Autodesk Inventor part; units mm, degrees
ref_plane "Work Plane1" through (3, 0, 1) normal (0, 0, 1) x (1, 0, 0)
ref_plane "YZ Plane" through (0, 0, 0) normal (1, 0, 0) x (0, 1, 0)
ref_plane "XZ Plane" through (0, 0, 0) normal (0, 1, 0) x (-1, 0, 0)
sketch "Sketch1" plane through (0, 0, 0) normal (0, 1, 0) x (-1, 0, 0)
  line L0 (0, 0) -> (-6, 0)
  line L1 (-6, 0) -> (-6, -9)
  line L2 (-6, -9) -> (0, -9)
  line L3 (0, -9) -> (0, 0)
  dimension "d0" = 6
  dimension "d1" = 9
extrude "Extrusion1" add sketch "Sketch1" along normal blind 6
sketch "Sketch2" plane through (6, 0, -9) normal (0, 0, -1) x (-1, 0, 0)
  line L0 (0, 6) -> (6, 6)
  line L1 (0, 0) -> (6, 0)
  line L2 (1.5, 6) -> (4.5, 6)
  line L3 (4.5, 6) -> (4.5, 0)
  line L4 (4.5, 0) -> (1.5, 0)
  line L5 (1.5, 0) -> (1.5, 6)
  line L6 (0, 0) -> (0, 6)
  dimension "d4" = 3
  dimension "d5" = 1.5
sketch "Sketch3" plane through (0, 0, 0) normal (0, -1, 0) x (1, 0, 0)
  line L0 (6, 0) -> (6, -9)
  line L1 (0, 0) -> (6, 0)
  point P0 (3, 1)
  dimension "d6" = 3
  dimension "d7" = 1
ref_plane "Work Plane1" through (3, 0, 1) normal (0, 0, 1) x (1, 0, 0)
sketch "Sketch4" plane through (3, 0, 1) normal (0, 0, 1) x (1, 0, 0)
  point P0 (-3, 0)
sketch "Sketch5" plane through (3, 0, 1) normal (0, 0, 1) x (1, 0, 0)
  circle A0 centre (0, 3) radius 1.5
  point P0 (-3, 0)
  dimension "d8" = 3
loft "Loft1" add profiles "Sketch5" section 1 edges at (3, 0, 0) (6, 3, 0) (3, 6, 0) (0, 3, 0)
extrude "Extrusion2" cut sketch "Sketch2" against normal blind 7 contours L0 L3 L1 L5
sketch "Sketch6" plane through (6, 0, -9) normal (1, 0, 0) x (0, 0, -1)
  line L0 (-9, 0) -> (-9, 6)
  line L1 (-9, 6) -> (0, 6)
  point P0 (-3, 3)
  dimension "d15" = 6
  dimension "d16" = 3
hole "Hole1" at (6, 3, -6) direction (-1, 0, 0) diameter 2.5 depth 1.5 tip angle 118
sketch "Sketch7" plane through (0, 0, -9) normal (-1, 0, 0) x (0, 0, 1)
  circle A0 centre (3, 3) radius 1.25
  point P0 (9, 0)
hole "Hole2" at (0, 3, -6) at (0, 3, -6) direction (1, 0, 0) diameter 3 depth 1.5 tip angle 118
thread "Thread1"
fillet "Fillet1" radius 3 4 edges at (5.25, 6, -9) (5.25, 0, -9) (0.75, 0, -9) (0.75, 6, -9)
sketch "Sketch8" plane through (6, 0, -2) normal (0, 0, -1) x (-1, 0, 0)
  line L0 (4.5, 6) -> (4.5, 0)
  line L1 (1.5, 6) -> (4.5, 6)
  line L2 (1.5, 0) -> (1.5, 6)
  line L3 (4.5, 0) -> (1.5, 0)
  point P0 (6, 0)
  point P1 (3, 3)
properties material "Brass, Soft Yellow, Welded"
Input: part model. Units: mm. Frame: model coordinates. A direction names the side the tool comes from. Coordinates: 2 decimals unless noted, no trailing zeros. Order: outer loops, then holes, each group sorted by start corner. A loop starts at its lowest first (then second) coordinate and runs counter-clockwise, first axis right, second up. Notation, with made-up numbers: M -20.75,70 L -6.75,70 A24 ccw -6.75,97 Z; hole C 49,86.25 d5. An arc over 180 degrees is marked long. Write item = value, one per line. Start each with the question number.
(1) Line query: line 1 along X through (y, z) = (0.75, -5.75); line 2 along Y through (x, z) = (5.2, -6). Output: solid intervals per line, ascending. Write a range as [from, to].
(2) First-contact query: P1, Ø2, axis at y = 3, z = -6, coming from the +X side; P2, Ø1.5, axis at x = 3.5, y = 3, coming from the -Z side. Flat tips, straight axial feed; report the tip coordinate or a pass-through.
(3) Reachability of faces 5 (the flat face through (1.5, 3, -4)), 6 (the cylindrical face through (0.74, 0.9, -8.14)) from +Z, -Z, +X, -X, +Y, -Y: full face, straight path, thin tool, end or side. Return the list, or none.
(4) Pull-direction query (Y, two-part tool) for faces 1 (the cylindrical face through (5.24, 2.95, -4.75)), 2 (the flat face through (3, 6, -1.6)), 3 (the cylindrical face through (0.76, 1.99, -7.11)), 4 (the flat face through (3, 3, -2)); classes: released by +Y, released by -Y, zero draft, split by the parting line, or undercut.
(5) Section B-B on y = 3.5. Give the number of separate pieces and of enclosed holes in the cut face, and give its area (3 significant figures).
(6) Section A-A on z = -3.75. Output: boundary loops of the cut face in (x, y).
Result set:
q1.line_1 = [0, 1.5], [4.5, 6]
q1.line_2 = [0, 1.75], [4.25, 6]
q2.P1 = through
q2.P2 = -2
q3.face_5 = -Z, +Y, -Y
q3.face_6 = -Z, +X, -X, -Y
q4.face_1 = undercut
q4.face_2 = released by +Y
q4.face_3 = undercut
q4.face_4 = zero draft
q5.separate_pieces = 3
q5.enclosed_holes = 0
q5.area = 29.7 mm²
q6.outline = M 0,0 L 1.5,0 L 1.5,6 L 0,6 Z; M 4.5,0 L 6,0 L 6,6 L 4.5,6 Z
